Here's how the part is built. I have some questions about the finished solid (model axes, mm). Face numbers are marked on the shaded views. A direction names the side the tool comes from. Coordinates: 2 decimals unless noted, no trailing zeros. Loops run counter-clockwise (first coordinate to the right, second up) from the corner with the lowest first, then second, coordinate; pieces in that order, holes last. Notation, with made-up numbers: M 69,-16.5 L 96,-16.5 A32 ccw 96,14.5 Z; hole C 14.25,49 d2. An arc over 180 degrees is marked long. Use CSV: the item, a comma, the result in double quotes. Start each with the question number.
Q1. Which directions (+Z, -Z, +X, -X, +Y, -Y) give clear straight access to the entire face, cutting with the end or side of a thin tool? Please do the marked faces 5, 6 and 7.
Q2. If we section it at C-C (z = 7.5): Please give me the cut outline in (x, y).
Q3. If we section it at D-D (x = 10.75): Please give me the cut outline in (y, z).
Q4. Please list where these lines run through material, in increasing order: probe 1 along X at (y, z) = (30, 12.25); probe 2 along Y at (x, z) = (8, 14.25); probe 3 along Y at (x, z) = (17.25, 10.25). Write a range as [from, to].
Q5. If we mould it in two halves opening along X, with no side actions, what happens to the marked faces 1, 2, 3 and 4? For each: +X half, -X half, draft (parallel to the pull), parting line (faces both ways), or undercut.
Q6. If we section it at A-A (y = 40.64): Please give me the cut outline in (x, z).
Q7. If we section it at B-B (y = 20): Please give me the cut outline in (x, z).
Q8. For pin 1 Ø3 at (y, z) = (-10.5, 5.5) entering from -X; pin 2 Ø1 at (x, z) = (4.5, 15.5) entering from +Y; pin 3 Ø1.5 at (x, z) = (5, 4) entering from -Y, each with a flat end and sliding along its axis, tell me the tip position at first contact or that it passes through.
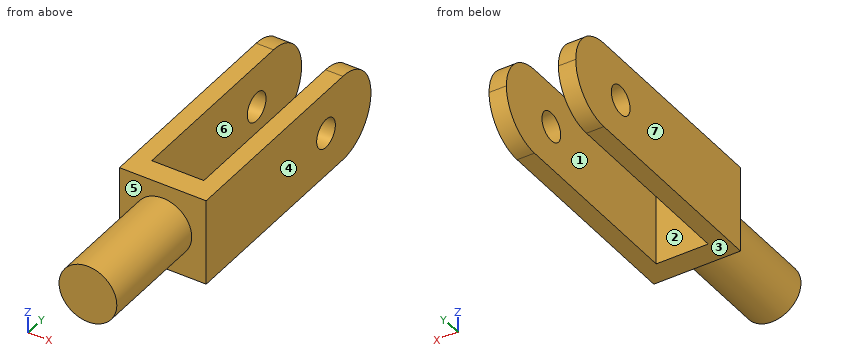
from build123d import *

# Parameters (mm, degrees)
SKETCH1_W           = 19.05
SKETCH1_H           = 19.05
BOSS_EXTRUDE1_DEPTH = 5.08
SKETCH2_W           = 3.81
SKETCH2_H           = 19.05
BOSS_EXTRUDE2_DEPTH = 50.8
FILLET1_R           = 9.525
SKETCH3_R           = 3.175
CUT_EXTRUDE1_DEPTH  = 63.035307688
SKETCH4_R           = 6.35
BOSS_EXTRUDE3_DEPTH = 25.4


with BuildPart() as part:
    # Sketch1 → Boss-Extrude1 (new body)
    with BuildSketch(Plane(origin=(0, 0, 0), x_dir=(1, 0, 0), z_dir=(0, 1, 0))):
        with Locations((9.525, -9.525)):
            Rectangle(SKETCH1_W, SKETCH1_H)
    extrude(amount=BOSS_EXTRUDE1_DEPTH)

    # Sketch2 → Boss-Extrude2 (add)
    with BuildSketch(Plane(origin=(0, 5.08, 0), x_dir=(1, 0, 0), z_dir=(0, 1, 0))):
        with Locations((1.905, -9.525)):
            Rectangle(SKETCH2_W, SKETCH2_H)
        with Locations((17.145, -9.525)):
            Rectangle(SKETCH2_W, SKETCH2_H)
    extrude(amount=BOSS_EXTRUDE2_DEPTH)

    # Fillet1
    fillet1_edges = [part.edges().sort_by_distance(p)[0] for p in [
        (1.905, 55.88, 0),
        (17.145, 55.88, 0),
        (1.905, 55.88, 19.05),
        (17.145, 55.88, 19.05),
    ]]
    fillet(fillet1_edges, radius=FILLET1_R - 0.0001)  # a hair under: the kernel refuses the full size

    # Sketch3 → Cut-Extrude1 (cut, through all)
    with BuildSketch(Plane.ZY):
        with Locations((9.525, 40.64)):
            Circle(SKETCH3_R)
    extrude(amount=-CUT_EXTRUDE1_DEPTH, mode=Mode.SUBTRACT)

    # Sketch4 → Boss-Extrude3 (add)
    with BuildSketch(Plane.XZ):
        with Locations(Location((9.525, 9.525, 0), (0, 0, 270))):
            Circle(SKETCH4_R)
    extrude(amount=BOSS_EXTRUDE3_DEPTH)


solid = part.part
Results below:
1,face 5,"-Y"
1,face 6,"+Z, -Z, +Y"
1,face 7,"+Z, -Z, -X, +Y, -Y"
2,outline,"M 0,0 L 3.51,0 L 3.51,-25.4 L 15.54,-25.4 L 15.54,0 L 19.05,0 L 19.05,38.19 L 15.24,38.19 L 15.24,5.08 L 3.81,5.08 L 3.81,38.19 L 0,38.19 Z; M 0,43.09 L 3.81,43.09 L 3.81,55.66 L 0,55.66 Z; M 15.24,43.09 L 19.05,43.09 L 19.05,55.66 L 15.24,55.66 Z"
3,outline,"M -25.4,3.29 L 0,3.29 L 0,0 L 5.08,0 L 5.08,19.05 L 0,19.05 L 0,15.76 L -25.4,15.76 Z"
4,probe 1,"[0, 3.81], [15.24, 19.05]"
4,probe 2,"[-25.4, 5.08]"
4,probe 3,"[0, 37.55], [43.73, 55.85]"
5,face 1,"undercut"
5,face 2,"undercut"
5,face 3,"draft"
5,face 4,"+X half"
6,outline,"M 0,0 L 3.81,0 L 3.81,6.35 L 0,6.35 Z; M 0,12.7 L 3.81,12.7 L 3.81,19.05 L 0,19.05 Z; M 15.24,0 L 19.05,0 L 19.05,6.35 L 15.24,6.35 Z; M 15.24,12.7 L 19.05,12.7 L 19.05,19.05 L 15.24,19.05 Z"
7,outline,"M 0,0 L 3.81,0 L 3.81,19.05 L 0,19.05 Z; M 15.24,0 L 19.05,0 L 19.05,19.05 L 15.24,19.05 Z"
8,pin 1,"x = 3.7"
8,pin 2,"y = 5.08"
8,pin 3,"y = 0"
